```python
from build123d import *

# Parameters (mm, degrees)
SKETCH1_W                    = 45
SKETCH1_H                    = 32
BOSS_EXTRUDE1_DEPTH          = 12
SKETCH2_W                    = 45
SKETCH2_H                    = 10.5
CUT_EXTRUDE1_DEPTH           = 4.5
SKETCH3_R                    = 1.5
CUT_EXTRUDE2_DEPTH           = 7.5
SKETCH4_R                    = 6.35
CUT_EXTRUDE3_DEPTH           = 12
SKETCH5_W                    = 15
SKETCH5_H                    = 6.5
BOSS_EXTRUDE3_DEPTH          = 10
SKETCH6_W                    = 15
SKETCH6_H                    = 6.5
BOSS_EXTRUDE4_DEPTH          = 10
SKETCH7_W                    = 2
SKETCH7_H                    = 5
BOSS_EXTRUDE5_DEPTH          = 4
M2_5X0_45_TAPPED_HOLE1_D     = 2.05
M2_5X0_45_TAPPED_HOLE1_DEPTH = 11.499
M2_5X0_45_TAPPED_HOLE1_TIP   = 0.615882135
CUT_EXTRUDE4_REACH           = 65.6
CUT_EXTRUDE4_END_RADIUS      = 6.35
SKETCH10_R                   = 1.025
FILLET1_DEPTH                = 11
FILLET2_R                    = 2
FILLET3_DEPTH                = 11
FILLET4_R                    = 2
FILLET5_START                = -43
FILLET5_DEPTH                = 11
FILLET6_START                = -43
FILLET6_DEPTH                = 11
FILLET7_R                    = 2
CUT_EXTRUDE5_REACH           = 60.215
FILLET8_R                    = 2


with BuildPart() as part:
    # Sketch1 → Boss-Extrude1 (new body)
    with BuildSketch(Plane(origin=(0, 0, 0), x_dir=(1, 0, 0), z_dir=(0, 1, 0))):
        with Locations((22.5, 16)):
            Rectangle(SKETCH1_W, SKETCH1_H)
    extrude(amount=BOSS_EXTRUDE1_DEPTH)

    # Sketch2 → Cut-Extrude1 (cut)
    with BuildSketch(Plane(origin=(0, 12, 0), x_dir=(1, 0, 0), z_dir=(0, 1, 0))):
        with Locations((22.5, 26.75)):
            Rectangle(SKETCH2_W, SKETCH2_H)
    extrude(amount=-CUT_EXTRUDE1_DEPTH, mode=Mode.SUBTRACT)

    # Sketch3 → Cut-Extrude2 (cut)
    with BuildSketch(Plane(origin=(0, 7.5, 0), x_dir=(1, 0, 0), z_dir=(0, 1, 0))):
        with Locations(Location((22.5, 27, 0), (0, 0, 270))):
            Circle(SKETCH3_R)
    extrude(amount=-CUT_EXTRUDE2_DEPTH, mode=Mode.SUBTRACT)

    # Sketch4 → Cut-Extrude3 (cut)
    with BuildSketch(Plane(origin=(0, 12, 0), x_dir=(1, 0, 0), z_dir=(0, 1, 0))):
        with Locations(Location((22.5, 11.5, 0), (0, 0, 270))):
            Circle(SKETCH4_R)
    extrude(amount=-CUT_EXTRUDE3_DEPTH, mode=Mode.SUBTRACT)

    # Sketch5 → Boss-Extrude3 (add)
    with BuildSketch(Plane(origin=(0, 0, -32), x_dir=(-1, 0, 0), z_dir=(0, 0, -1))):
        with Locations((-37.5, 3.25)):
            Rectangle(SKETCH5_W, SKETCH5_H)
        with Locations((-7.5, 3.25)):
            Rectangle(SKETCH5_W, SKETCH5_H)
    extrude(amount=BOSS_EXTRUDE3_DEPTH)

    # Sketch6 → Boss-Extrude4 (add)
    with BuildSketch(Plane.XY):
        with Locations((7.5, 3.25)):
            Rectangle(SKETCH6_W, SKETCH6_H)
        with Locations((37.5, 3.25)):
            Rectangle(SKETCH6_W, SKETCH6_H)
    extrude(amount=BOSS_EXTRUDE4_DEPTH)

    # Sketch7 → Boss-Extrude5 (add)
    with BuildSketch(Plane(origin=(0, 12, 0), x_dir=(1, 0, 0), z_dir=(0, 1, 0))):
        with Locations((9, 10.75)):
            Rectangle(SKETCH7_W, SKETCH7_H)
        with Locations((36, 10.75)):
            Rectangle(SKETCH7_W, SKETCH7_H)
    extrude(amount=BOSS_EXTRUDE5_DEPTH)

    # M2.5x0.45 Tapped Hole1
    with Locations(Plane.XY):
        with Locations((22.5, 8.5)):
            Hole(M2_5X0_45_TAPPED_HOLE1_D / 2, depth=M2_5X0_45_TAPPED_HOLE1_DEPTH)
            with Locations((0, 0, -(M2_5X0_45_TAPPED_HOLE1_DEPTH + M2_5X0_45_TAPPED_HOLE1_TIP / 2))):  # 118° drill point
                Cone(0, M2_5X0_45_TAPPED_HOLE1_D / 2, M2_5X0_45_TAPPED_HOLE1_TIP, mode=Mode.SUBTRACT)

    # Cut-Extrude4: up to this cylinder (the profile starts outside it)
    cut_extrude4_end = Plane(origin=(22.5, 4, -11.5), z_dir=(0, 1, 0)) * Cylinder(CUT_EXTRUDE4_END_RADIUS, 144.9, mode=Mode.PRIVATE)
    # Sketch10 → Cut-Extrude4 (cut, up to the surface)
    with BuildSketch(Plane.XY, mode=Mode.PRIVATE) as cut_extrude4_sk1:
        with Locations((22.5, 4)):
            Circle(SKETCH10_R)
    cut_extrude4_tool1 = extrude(cut_extrude4_sk1.sketch, amount=-CUT_EXTRUDE4_REACH, mode=Mode.PRIVATE) - cut_extrude4_end
    add(cut_extrude4_tool1.solids().sort_by_distance((22.5, 4, 0))[0], mode=Mode.SUBTRACT)

    # Fillet1: read off the stored shape, not the designer's step
    # Fillet1 outline → Fillet1 (cut)
    with BuildSketch(Plane.XY):
        with BuildLine():
            Line((0, 0), (2, 0))
            ThreePointArc((2, 0), (0.585786438, 0.585786438), (0, 2))
            Line((0, 2), (0, 0))
        make_face()
    extrude(amount=FILLET1_DEPTH, mode=Mode.SUBTRACT)

    # Fillet2
    fillet2_edges = [part.edges().sort_by_distance(p)[0] for p in [
        (15, 0, 5),
        (30, 0, 5),
    ]]
    fillet(fillet2_edges, radius=FILLET2_R)

    # Fillet3: read off the stored shape, not the designer's step
    # Fillet3 outline → Fillet3 (cut)
    with BuildSketch(Plane.XY):
        with BuildLine():
            ThreePointArc((45, 2), (44.414213562, 0.585786438), (43, 0))
            Line((43, 0), (45, 0))
            Line((45, 0), (45, 2))
        make_face()
    extrude(amount=FILLET3_DEPTH, mode=Mode.SUBTRACT)

    # Fillet4
    fillet4_edges = [part.edges().sort_by_distance(p)[0] for p in [
        (30, 0, -37),
        (15, 0, -37),
    ]]
    fillet(fillet4_edges, radius=FILLET4_R)

    # Fillet5: read off the stored shape, not the designer's step
    # Fillet5 outline → Fillet5 (cut)
    with BuildSketch(Plane.XY.offset(FILLET5_START)):
        with BuildLine():
            ThreePointArc((45, 2), (44.414213562, 0.585786438), (43, 0))
            Line((43, 0), (45, 0))
            Line((45, 0), (45, 2))
        make_face()
    extrude(amount=FILLET5_DEPTH, mode=Mode.SUBTRACT)

    # Fillet6: read off the stored shape, not the designer's step
    # Fillet6 outline → Fillet6 (cut)
    with BuildSketch(Plane.XY.offset(FILLET6_START)):
        with BuildLine():
            Line((0, 0), (2, 0))
            ThreePointArc((2, 0), (0.585786438, 0.585786438), (0, 2))
            Line((0, 2), (0, 0))
        make_face()
    extrude(amount=FILLET6_DEPTH, mode=Mode.SUBTRACT)

    # Fillet7
    fillet7_edges = [part.edges().sort_by_distance(p)[0] for p in [
        (45, 6.5, -37),
        (30, 6.5, -37),
        (15, 6.5, -37),
        (0, 6.5, -37),
        (0, 6.5, 5),
        (15, 6.5, 5),
        (45, 6.5, 5),
        (30, 6.5, 5),
    ]]
    fillet(fillet7_edges, radius=FILLET7_R)

    # Cut-Extrude5: up to this face of the body (flat: up to its plane)
    cut_extrude5_end = Plane(part.part.faces().sort_by_distance((8, 14, -10.75))[0])
    # Sketch11 → Cut-Extrude5 (cut, up to the picked face)
    with BuildSketch(Plane(origin=(37, 0, 0), x_dir=(0, 0, -1), z_dir=(1, 0, 0)), mode=Mode.PRIVATE) as cut_extrude5_sk1:
        with BuildLine():
            Line((10, 14), (10, 12))
            Line((10, 12), (11.5, 12))
            Line((11.5, 12), (11.5, 14))
            ThreePointArc((11.5, 14), (10.75, 14.75), (10, 14))
        make_face()
    cut_extrude5_tool1 = split(extrude(cut_extrude5_sk1.sketch, amount=-CUT_EXTRUDE5_REACH, mode=Mode.PRIVATE), bisect_by=cut_extrude5_end, keep=Keep.BOTH, mode=Mode.PRIVATE)
    add(cut_extrude5_tool1.solids().sort_by(Axis((37, 13.299936, -10.75), (-1, 0, 0)))[0], mode=Mode.SUBTRACT)

    # Fillet8
    fillet8_edges = [part.edges().sort_by_distance(p)[0] for p in [
        (36, 12, -13.25),
        (9, 12, -8.25),
        (9, 12, -13.25),
        (36, 12, -8.25),
    ]]
    fillet(fillet8_edges, radius=FILLET8_R)


solid = part.part
```
Part model, mm, in its own coordinate system. A direction names the side the tool comes from. Coordinates: 2 decimals unless noted, no trailing zeros. Write each loop counter-clockwise with the first axis right and the second up, starting at its lowest first coordinate (ties: lowest second). Pieces come first, ordered by that corner, then holes.
Item 1: Pin check, flat tips, straight feed: pin 1 (10 mm diameter, centred on x = 17, z = -7.5, fed in from +Y); pin 2 (0.6 mm diameter, centred on x = 9, y = 14.5, fed in from +Z); pin 3 (1.6 mm diameter, centred on x = 36, y = 12.5, fed in from +Z); pin 4 (10 mm diameter, centred on x = 22.5, z = -11.5, fed in from +Y). Stop position of each tip, or through.
Item 2: Slice it at C-C (x = 22.5). Write the cut outline in (y, z) (3 decimals), and give its area (3 significant figures).
Item 3: Probe line 1 (X direction, y = 2, z = -27); line 2 (X direction, y = 8, z = -11.5); line 3 (Z direction, x = 6, y = 8.75). List the from-to ranges inside material, lowest first.
Item 4: Slice it at B-B (y = 8.5). Write the cut outline in (x, z) (3 decimals), and give its area (3 significant figures).
Item 5: Mould opens along Z. For faces 1 (the face through (23.51, 3.8, -28.11)), 2 (the face through (8, 3, -42)), 3 (the face through (44.43, 5.9, -37.07)) say: released by +Z, released by -Z, zero draft, split by the parting line, or undercut.
Item 6: Which spindle directions (+Z, -Z, +X, -X, +Y, -Y) get a long thin tool onto all of the face, cutting with end or side? Do faces 4 (the face through (8, 15, -11)), 5 (the face through (9, 15, -13.25)), 6 (the face through (14.43, 5.9, -37.07)), 7 (the face through (36, 13, -10)), 8 (the face through (0.4, 0.5, 0)). Say none if no direction does.
Item 7: Slice it at D-D (z = -10.75). Write the cut outline in (x, y).
Item 8: Slice it at A-A (z = -37). Write the cut outline in (x, y).
Results found:
1. pin 1: stops at y = 12
1. pin 2: stops at z = -8.25
1. pin 3: stops at z = 0
1. pin 4: passes through
2. outline: (0, -32) - (7.5, -32) - (7.5, -28.5) - (0, -28.5) - close; (0, -25.5) - (7.5, -25.5) - (7.5, -21.5) - (12, -21.5) - (12, -17.85) - (0, -17.85) - close; (0, -5.15) - (2.975, -5.15) - (2.975, 0) - (0, 0) - close; (5.025, -5.15) - (7.475, -5.15) - (7.475, 0) - (5.025, 0) - close; (9.525, -5.15) - (12, -5.15) - (12, 0) - (9.525, 0) - close
2. area: 141 mm2
3. line 1: x = 0 to 21, 24 to 45
3. line 2: x = 0 to 16.15, 28.85 to 45
3. line 3: z = -21.5 to 0
4. outline: (0, -21.5) - (45, -21.5) - (45, 0) - (23.525, 0) - (23.525, -5.233) arc R6.35 cw (long way) to (21.475, -5.233) - (21.475, 0) - (0, 0) - close
4. area: 830 mm2
5. face 1: undercut
5. face 2: released by -Z
5. face 3: zero draft
6. face 4: +Z, -Z, -X, +Y
6. face 5: -Z, +X, -X, +Y
6. face 6: -Z, +Y
6. face 7: +X, -X
6. face 8: +Z, -X, -Y
7. outline: (0, 0) - (16.19, 0) - (16.19, 12) - (0, 12) - close; (8, 14.75) - (10, 14.75) - (10, 16) - (8, 16) - close; (28.81, 0) - (45, 0) - (45, 12) - (28.81, 12) - close; (35, 14.75) - (37, 14.75) - (37, 16) - (35, 16) - close
8. outline: (0, 2) arc R2 ccw to (2, 0) - (13, 0) arc R2 ccw to (15, 2) - (15, 4.5) arc R2 ccw to (13, 6.5) - (2, 6.5) arc R2 ccw to (0, 4.5) - close; (30, 2) arc R2 ccw to (32, 0) - (43, 0) arc R2 ccw to (45, 2) - (45, 4.5) arc R2 ccw to (43, 6.5) - (32, 6.5) arc R2 ccw to (30, 4.5) - close
